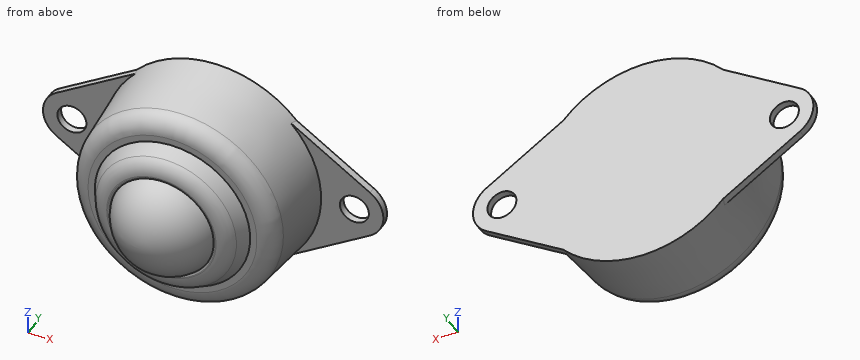
from build123d import *

# Parameters (mm, degrees)
FILLET1_R           = 2.5
SKETCH1_R           = 2
BOSS_EXTRUDE1_DEPTH = 1
FILLET2_R           = 0.25


with BuildPart() as part:
    # Sketch2 one side → Revolve1 (revolve)
    with BuildSketch(Plane.XY):
        with BuildLine():
            Line((0, -20), (0, -5))
            Line((0, -5), (0, 0))
            Line((0, 0), (-15, 0))
            Line((-15, 0), (-13.950136038, -12))
            Line((-13.950136038, -12), (-10.732050808, -12))
            Line((-10.732050808, -12), (-9, -15))
            Line((-9, -15), (-7.307879939, -15))
            Line((-7.307879939, -15), (-7.131103244, -14.823223305))
            ThreePointArc((-7.131103244, -14.823223305), (-4.406008694, -18.569356423), (0, -20))
        make_face()
    revolve(axis=Axis((0, 0, 0), (0, -1, 0)))

    # Fillet1
    fillet1_edges = [part.edges().sort_by_distance(p)[0] for p in [
        (9, -15, 0),
        (13.950136038, -12, 0),
    ]]
    fillet(fillet1_edges, radius=FILLET1_R)

    # Sketch1 → Boss-Extrude1 (add)
    # profile 1 of 2: a face of its own
    with BuildSketch(Plane(origin=(0, 0, 0), x_dir=(1, 0, 0), z_dir=(0, 1, 0))):
        with BuildLine():
            ThreePointArc((-21.653846154, 3.370600354), (-23.5, 0), (-21.653846154, -3.370600354))
            Line((-21.653846154, -3.370600354), (-7.807692308, -12.218426283))
            ThreePointArc((-7.807692308, -12.218426283), (-14.5, 0), (-7.807692308, 12.218426283))
            Line((-7.807692308, 12.218426283), (-21.653846154, 3.370600354))
        make_face()
        with Locations(Location((-19.5, 0, 0), (0, 0, 270))):
            Circle(SKETCH1_R, mode=Mode.SUBTRACT)
    # profile 2 of 2: a face of its own
    with BuildSketch(Plane(origin=(0, 0, 0), x_dir=(1, 0, 0), z_dir=(0, 1, 0))):
        with BuildLine():
            Line((21.653846154, 3.370600354), (7.807692308, 12.218426283))
            ThreePointArc((7.807692308, 12.218426283), (14.5, 0), (7.807692308, -12.218426283))
            Line((7.807692308, -12.218426283), (21.653846154, -3.370600354))
            ThreePointArc((21.653846154, -3.370600354), (23.5, 0), (21.653846154, 3.370600354))
        make_face()
        with Locations(Location((19.5, 0, 0), (0, 0, 270))):
            Circle(SKETCH1_R, mode=Mode.SUBTRACT)
    extrude(amount=-BOSS_EXTRUDE1_DEPTH)

    # Fillet2
    fillet2_edges = [part.edges().sort_by_distance(p)[0] for p in [
        (7.307879939, -15, 0),
    ]]
    fillet(fillet2_edges, radius=FILLET2_R)


solid = part.part
The listing builds one solid part. Answer for the finished solid, in the listing's coordinates (mm). Give positions to 0.01 mm unless a question says otherwise; leave off trailing zeros. Loops run counter-clockwise (first coordinate to the right, second up) from the corner with the lowest first, then second, coordinate; pieces in that order, holes last. Notation, with made-up numbers: (42.5, -36) - (85.5, -36) arc R13 ccw to (85.5, -28) - close; hole circle Ø2 at (55.25, -38.75). An arc over 180 degrees is marked (long way). Answer as a JSON object with one key per item and string values.
1. Flat-ended cylindrical pins translate along their axes: pin 1 Ø5 at (x, y) = (-14, -3) entering from +Z; pin 2 Ø5 at (x, z) = (16.5, -11.5) entering from -Y; pin 3 Ø12 at (y, z) = (-7, 10) entering from -X; pin 4 Ø14 at (x, z) = (-16.5, -4.5) entering from -Y. Find the tip coordinate at first contact, or state that the pin passes through.
Determined:
{"pin 1": "z = 9.24", "pin 2": "through", "pin 3": "x = -13.9", "pin 4": "y = -13.09"}
2. A cutting plane is placed at A-A (z = 0). Give the number of separate pieces and of enclosed holes in the cut face, then the cut area to 3 significant figures.
Determined:
{"separate pieces": "3", "enclosed holes": "0", "area": "464 mm²"}
3. A cutting plane is placed at C-C (y = -17.5). Write down the section's boundary in (x, z).
Determined:
{"outline": "circle Ø11.18 at (0, 0)"}
4. A cutting plane is placed at D-D (y = -2). Write down the section's boundary in (x, z), then the cut area to 3 significant figures.
Determined:
{"outline": "circle Ø29.65 at (0, 0)", "area": "690 mm²"}
5. Find the intervals of material crossed by L1, parallel to X at y = -0.5, z = 0; L2, parallel to X at y = -13.75, z = 6.5; L3, parallel to Y at x = -16, z = -6.5, in increasing order. Write a range as [from, to].
Determined:
{"L1": "[-23.5, -21.5], [-17.5, 17.5], [21.5, 23.5]", "L2": "[-7.23, 7.23]", "L3": "[-1, 0]"}
6. A cutting plane is placed at B-B (x = -19.5). Write down the section's boundary in (y, z), then the cut area to 3 significant figures.
Determined:
{"outline": "(-1, -4.75) - (0, -4.75) - (0, -2) - (-1, -2) - close; (-1, 2) - (0, 2) - (0, 4.75) - (-1, 4.75) - close", "area": "5.49 mm²"}
